For this review, use the dimensioned drawing (mm, ordinates from the lowest corner) and the shaded views. A direction names the side the tool comes from. Give positions to 0.01 mm unless a question says otherwise; leave off trailing zeros. Loops run counter-clockwise (first coordinate to the right, second up) from the corner with the lowest first, then second, coordinate; pieces in that order, holes last. Notation, with made-up numbers: (59.25, 45.25) -> (93.25, 45.25) arc R18 cw to (93.25, 52.25) -> close; hole circle Ø9 at (65.25, 37.5). An arc over 180 degrees is marked (long way). Use a Markdown table: item, result. Add a question column.
1. For the marked faces 5 and 6, list the 3-axis set-ups (+Z, -Z, +X, -X, +Y, -Y) from which the entire face can be reached by the end or side of a thin tool; tool diameter is ignored.
2. Add section B-B (z = 3.5). State the section outline as (x, y) points, and give its area (4 significant figures).
3. Add section A-A (x = 3.5). State the section outline as (y, z) points, and give its area (3 significant figures).
4. Draft analysis for pull direction X (two halves, no side actions). For the marked faces 1, 2, 3 and 4, state which applies: pulls with the +X half, pulls with the -X half, needs draft (parallel to the pull), parting line crosses it, or undercut.
5. Add section D-D (z = 5.5). State the section outline as (x, y) points.
6. To check wall thickness, follow line 1 (X direction, y = 0.4, z = 3.5); line 2 (Z direction, x = 3.5, y = 1.75); line 3 (X direction, y = 1.7, z = 4). State the ranges of each line that lie inside material, in increasing order.
7. Add section C-C (y = 2.7). State the section outline as (x, z) points, and give its area (3 significant figures).
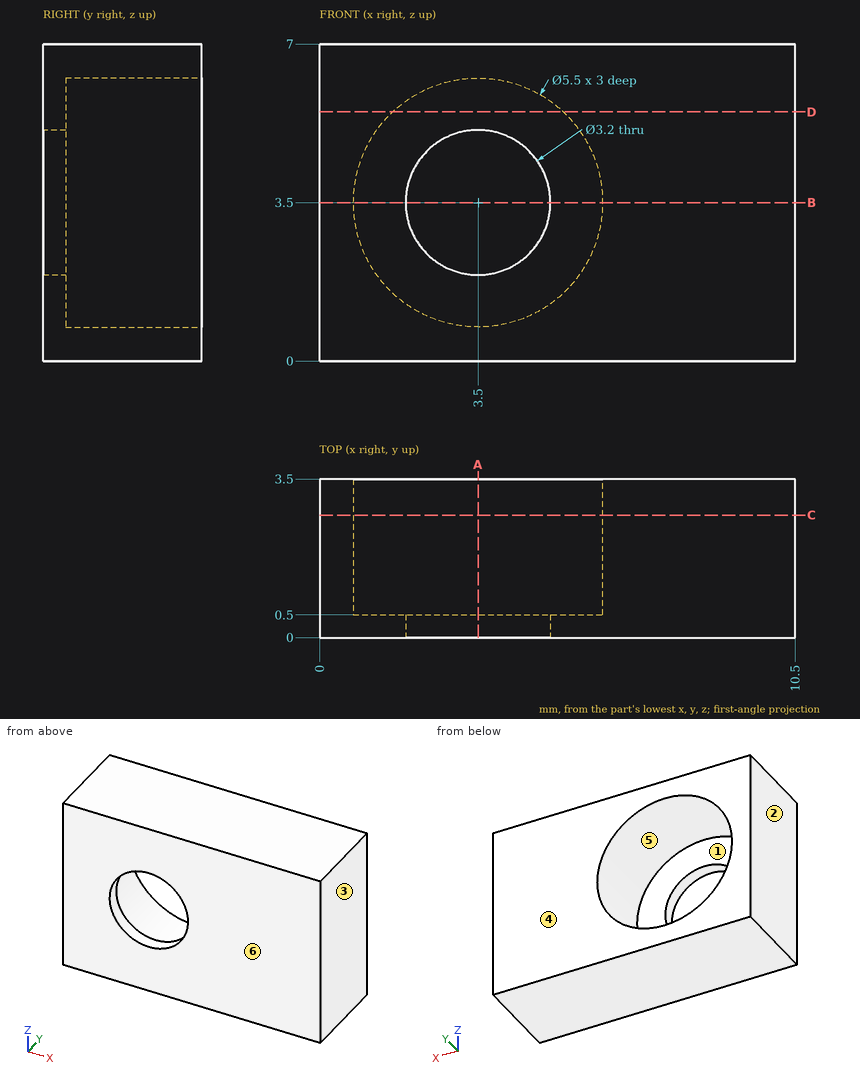
Taken from the geometry:
| question | item | result |
|---|---|---|
| 1 | face 5 | +Y |
| 1 | face 6 | +Z, -Z, +X, -X, -Y |
| 2 | outline | (0, 0) -> (1.9, 0) -> (1.9, 0.5) -> (0.75, 0.5) -> (0.75, 3.5) -> (0, 3.5) -> close; (5.1, 0) -> (10.5, 0) -> (10.5, 3.5) -> (6.25, 3.5) -> (6.25, 0.5) -> (5.1, 0.5) -> close |
| 2 | area | 18.65 mm^2 |
| 3 | outline | (0, 0) -> (3.5, 0) -> (3.5, 0.75) -> (0.5, 0.75) -> (0.5, 1.9) -> (0, 1.9) -> close; (0, 5.1) -> (0.5, 5.1) -> (0.5, 6.25) -> (3.5, 6.25) -> (3.5, 7) -> (0, 7) -> close |
| 3 | area | 6.40 mm^2 |
| 4 | face 1 | undercut |
| 4 | face 2 | pulls with the -X half |
| 4 | face 3 | pulls with the +X half |
| 4 | face 4 | needs draft |
| 5 | outline | (0, 0) -> (10.5, 0) -> (10.5, 3.5) -> (5.39, 3.5) -> (5.39, 0.5) -> (1.61, 0.5) -> (1.61, 3.5) -> (0, 3.5) -> close |
| 6 | line 1 | x = 0 to 1.9, 5.1 to 10.5 |
| 6 | line 2 | z = 0 to 0.75, 6.25 to 7 |
| 6 | line 3 | x = 0 to 0.8, 6.2 to 10.5 |
| 7 | outline | (0, 0) -> (10.5, 0) -> (10.5, 7) -> (0, 7) -> close; hole circle Ø5.5 at (3.5, 3.5) |
| 7 | area | 49.7 mm^2 |
